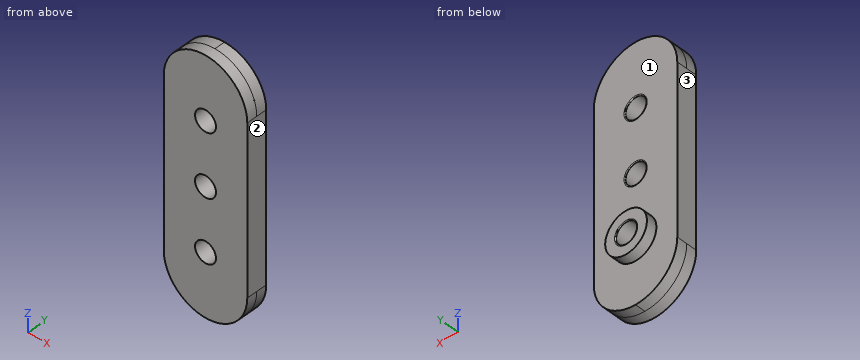
Autodesk Inventor part; units mm, degrees
ref_plane "YZ Plane" through (0, 0, 0) normal (1, 0, 0) x (0, 1, 0)
ref_plane "XZ Plane" through (0, 0, 0) normal (0, 1, 0) x (-1, 0, 0)
ref_plane "XY Plane" through (0, 0, 0) normal (0, 0, 1) x (1, 0, 0)
sketch "Sketch1" plane through (0, 0, 0) normal (0, 1, 0) x (-1, 0, 0)
  line L0 (0, 0) -> (25.4, 0)
  line L1 (25.4, 0) -> (25.4, -76.2)
  line L2 (25.4, -76.2) -> (0, -76.2)
  line L3 (0, -76.2) -> (0, 0)
  dimension "d0" = 25.4
  dimension "d1" = 76.2
extrude "Extrusion1" add sketch "Sketch1" along normal blind 3.175
sketch "Sketch2" plane through (0, 3.175, 0) normal (0, 1, 0) x (1, 0, 0)
  line L0 (-25.4, 76.2) -> (-25.4, 0)
  line L1 (0, 76.2) -> (-25.4, 76.2)
  line L2 (-25.4, 0) -> (0, 76.2)
  line L3 (0, 76.2) -> (-25.4, 76.2)
  line L4 (-25.4, 76.2) -> (0, 0)
  line L5 (0, 0) -> (-12.7, 38.1)
  line L6 (-25.4, 0) -> (0, 0)
  line L7 (-12.7, 0) -> (-12.7, 76.2)
  circle A0 centre (-12.7, 38.1) radius 3.175
  line L8 (-12.7, 38.1) -> (-12.7, 0)
  circle A1 centre (-12.7, 19.05) radius 3.175
  line L9 (-12.7, 38.1) -> (-12.7, 76.2)
  circle A2 centre (-12.7, 57.15) radius 3.175
  dimension "d4" = 6.35
  dimension "d5" = 6.35
  dimension "d6" = 6.35
extrude "Extrusion2" cut sketch "Sketch2" against normal blind 3.175 contours A0 L7 L4 | L4 L2 A0 | L2 L7 A0 | A2 L7 | L7 A2 | L7 A0 L2 | L2 A0 L4 | L4 A0 L7 | A1 L7 | L7 A1
fillet "Fillet1" radius 12.7 4 edges at (0, 1.5875, 0) (-25.4, 1.5875, 0) (0, 1.5875, -76.2) (-25.4, 1.5875, -76.2)
fillet "Fillet2" radius 0.3175 3 edges at (-15.875, 3.175, -57.15) (-15.875, 3.175, -38.1) (-15.875, 3.175, -19.05)
sketch "Sketch3" plane through (0, 3.175, 0) normal (0, 1, 0) x (1, 0, 0)
  circle A0 centre (-12.7, 57.15) radius 3.175
  circle A1 centre (-12.7, 57.15) radius 6.35
  point P0 (0, 0)
  dimension "d11" = 12.7
extrude "Extrusion3" add sketch "Sketch3" along normal blind 3.175
sketch "Sketch4" plane through (-12.7, 6.35, -57.15) normal (0, 1, 0) x (1, 0, 0)
  circle A0 centre (0, 0) radius 6.35
  circle A1 centre (0, 0) radius 3.175
  point P0 (12.7, -57.15)
extrude "Extrusion4" add sketch "Sketch4" against normal through all
fillet "Fillet3" radius 0.3175 1 edges at (-15.875, 6.35, -57.15)
sketch "Sketch5" plane through (0, 0, 0) normal (0, -1, 0) x (1, 0, 0)
  circle A0 centre (-12.7, -38.1) radius 3.175
  circle A1 centre (-12.7, -19.05) radius 3.175
  arc A2 (-25.4, -63.5) -> (0, -63.5) centre (-12.7, -63.5) ccw
  line L0 (0, -12.7) -> (0, -63.5)
  arc A3 (0, -12.7) -> (-25.4, -12.7) centre (-12.7, -12.7) ccw
  line L1 (-25.4, -63.5) -> (-25.4, -12.7)
  circle A4 centre (-12.7, -57.15) radius 3.175
  point P0 (0, 0)
extrude "Extrusion5" add sketch "Sketch5" along normal blind 3.175
sketch "Sketch6" plane through (0, -3.175, 0) normal (0, -1, 0) x (1, 0, 0)
  line L0 (-25.4, -12.7) -> (-25.4, -63.5)
  arc A0 (-25.4, -63.5) -> (0, -63.5) centre (-12.7, -63.5) ccw
  line L1 (0, -63.5) -> (0, -12.7)
  arc A1 (0, -12.7) -> (-25.4, -12.7) centre (-12.7, -12.7) ccw
  circle A2 centre (-12.7, -57.15) radius 3.175
  circle A3 centre (-12.7, -19.05) radius 3.175
  circle A4 centre (-12.7, -38.1) radius 3.175
  circle A5 centre (-12.7, -57.15) radius 3.175
  circle A6 centre (-12.7, -57.15) radius 3.1877
  circle A7 centre (-12.7, -38.1) radius 3.175
  circle A8 centre (-12.7, -38.1) radius 3.175
  circle A9 centre (-12.7, -38.1) radius 3.1877
  circle A10 centre (-12.7, -19.05) radius 3.175
  circle A11 centre (-12.7, -19.05) radius 3.175
  circle A12 centre (-12.7, -19.05) radius 3.1877
  point P0 (0, 0)
  dimension "d19" = 6.3754
  dimension "d20" = 6.3754
  dimension "d21" = 6.3754
extrude "Extrusion6" cut sketch "Sketch6" against normal blind 25.4 contours A2 | A3 | A4 | A6 | A9 | A12
properties part number "Board"
The model under review builds one solid part; all positions refer to its coordinate system, in mm. Face numbers are marked on the shaded views. Round coordinates to 2 decimals unless told otherwise and drop trailing zeros.
1) Consider section B-B on y = 1.75. Give the number of separate pieces and of enclosed holes in the cut face, then the cut area to 3 significant figures.
Values follow:
separate pieces: 1
enclosed holes: 3
area: 1,700 mm2
2) Clearance check with flat-ended pins moving along their axes: P1, Ø2, axis at x = -6, z = -30.5, coming from the +Y side (3 decimals); P2, Ø5, axis at x = -12.7, z = -38.1, coming from the +Y side; P3, Ø3, axis at y = 5, z = -55, coming from the +X side. State where each tip first meets the part, or that it passes through.
Values follow:
P1: stops at y = 3.175
P2: passes through
P3: stops at x = -6.38
3) The part is to be moulded in two halves that separate along X. For the marked faces 1, 2 and 3, say which applies: pulls with the +X half, pulls with the -X half, needs draft (parallel to the pull), parting line crosses it, or undercut.
Values follow:
face 1: needs draft
face 2: pulls with the +X half
face 3: pulls with the -X half
4) Wall thickness on line 1 along Z through (x, y) = (-12.7, 0.25); line 2 along X through (y, z) = (1, -38.1); line 3 along X through (y, z) = (4, -57.15): over which ranges is each line inside the solid? List them lowest first.
Values follow:
line 1: z = -76.2 to -60.34, -53.96 to -41.29, -34.91 to -22.24, -15.86 to 0
line 2: x = -25.4 to -15.89, -9.51 to 0
line 3: x = -19.05 to -15.89, -9.51 to -6.35
